Check sheet for the modelled part. Datum: model origin and axes. Units: mm. Face numbers are marked on the shaded views. A direction names the side the tool comes from. Coordinates: 2 decimals unless noted, no trailing zeros. Loops run counter-clockwise (first coordinate to the right, second up) from the corner with the lowest first, then second, coordinate; pieces in that order, holes last. Notation, with made-up numbers: (-20, 12.25) - (11, 12.25) arc R10 cw to (11, 19.25) - close; hole circle Ø4 at (-3.5, 45). An arc over 180 degrees is marked (long way). Use a Markdown table: item, result. Add a question column.
1) Draft check along X on the marked faces 6, 7 and 8. Enter one of: pulls with the +X half, pulls with the -X half, needs draft (parallel to the pull), parting line crosses it, or undercut.
2) Sectioned sample at C-C, the plane x = 8.5. Enter the section's corners in (y, z).
3) Go/stop test with flat-tipped pins: P1, Ø1.5, axis at x = 9, y = 47.5, coming from the -Z side; P2, Ø6, axis at x = 15, z = 42, coming from the +Y side; P3, Ø6, axis at y = 72.5, z = 7.5, coming from the -X side. Record where each tip stops, or that it passes through.
4) Sectioned sample at B-B, the plane y = 18. Enter the section's corners in (x, z), then the cut area to 3 significant figures.
5) Sectioned sample at D-D, the plane z = 7.5. Enter the section's corners in (x, y).
6) Thickness scan on line 1 (Y direction, x = 13.5, z = 55.5); line 2 (X direction, y = 2.55, z = 62.5); line 3 (X direction, y = 77.5, z = 4.5). Record the ranges inside material, lowest first.
7) Sectioned sample at A-A, the plane z = 62.5. Enter the section's corners in (x, y), then the cut area to 3 significant figures.
8) Tool access check on the marked faces 1, 2, 3, 4 and 5. Record the directions out of +Z, -Z, +X, -X, +Y, -Y that give a thin tool (end or side, any length) a straight path to the whole face; none if there is none.
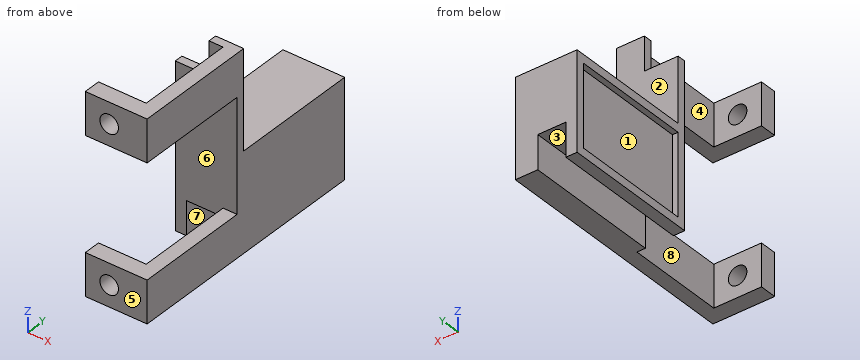
from build123d import *

# Parameters (mm, degrees)
SKETCH001_W  = 41
SKETCH001_H  = 40
PAD001_DEPTH = 22
SKETCH002_W  = 46
SKETCH002_H  = 35
PAD002_DEPTH = 22
SKETCH003_W  = 35
SKETCH003_H  = 17
PAD003_DEPTH = 70
SKETCH004_W  = 43
SKETCH004_H  = 29
PAD004_DEPTH = 2
SKETCH008_R  = 3.3
PAD006_DEPTH = 6
SKETCH007_R  = 3.3
PAD005_DEPTH = 6
SKETCH009_W  = 12
SKETCH009_H  = 12
PAD007_DEPTH = 3
SKETCH010_W  = 10
SKETCH010_H  = 49
PAD008_DEPTH = 12
SKETCH_W     = 90
SKETCH_H     = 70
PAD_DEPTH    = 22


with BuildPart() as body001:
    # Sketch001 (on Face1 of CopyPad) → Pad001 (new body)
    with BuildSketch(Plane.YZ.offset(22)):
        with Locations((20.5, 35)):
            Rectangle(SKETCH001_W, SKETCH001_H)
    extrude(amount=-PAD001_DEPTH)


with BuildPart() as body002:
    # Sketch002 (on Face1 of CopyPad001) → Pad002 (new body)
    with BuildSketch(Plane.YZ.offset(22)):
        with Locations((67, 52.5)):
            Rectangle(SKETCH002_W, SKETCH002_H)
    extrude(amount=-PAD002_DEPTH)


with BuildPart() as body003:
    # Sketch003 (on Face1 of CopyBoolean001) → Pad003 (new body)
    with BuildSketch(Plane.YX):
        with Locations((23.5, 8.5)):
            Rectangle(SKETCH003_W, SKETCH003_H)
    extrude(amount=-PAD003_DEPTH)


with BuildPart() as body004:
    # Sketch004 (on Face1 of CopyBoolean002) → Pad004 (new body)
    with BuildSketch(Plane(origin=(0, 0, 0), x_dir=(0, -1, 0), z_dir=(-1, 0, 0))):
        with Locations((-65.5, 17.5)):
            Rectangle(SKETCH004_W, SKETCH004_H)
    extrude(amount=-PAD004_DEPTH)


with BuildPart() as body007:
    # Sketch008 → Pad006 (new body)
    with BuildSketch(Plane(origin=(0, 0, 0), x_dir=(0, 0, -1), z_dir=(0, -1, 0))):
        with Locations((-7.5, 8.5)):
            Circle(SKETCH008_R)
    extrude(amount=-PAD006_DEPTH)


with BuildPart() as body007_1:
    # Body007 placement: moved
    add(body007.part.moved(Location((0, 0, 55))))


with BuildPart() as body006:
    # Sketch007 → Pad005 (new body)
    with BuildSketch(Plane(origin=(0, 0, 0), x_dir=(0, 0, -1), z_dir=(0, -1, 0))):
        with Locations((-7.5, 8.5)):
            Circle(SKETCH007_R)
    extrude(amount=-PAD005_DEPTH)


with BuildPart() as body008:
    # Sketch009 (on Face1 of CopyBoolean005) → Pad007 (new body)
    with BuildSketch(Plane.XZ.offset(-41)):
        with Locations((6, 64)):
            Rectangle(SKETCH009_W, SKETCH009_H)
    extrude(amount=-PAD007_DEPTH)


with BuildPart() as body009:
    # Sketch010 (on Face1 of CopyBoolean006) → Pad008 (new body)
    with BuildSketch(Plane(origin=(0, 0, 0), x_dir=(1, 0, 0), z_dir=(0, 0, -1))):
        with Locations((9, -65.5)):
            Rectangle(SKETCH010_W, SKETCH010_H)
    extrude(amount=-PAD008_DEPTH)


with BuildPart() as body:
    # Sketch → Pad (new body)
    with BuildSketch(Plane.YZ):
        with Locations((45, 35)):
            Rectangle(SKETCH_W, SKETCH_H)
    extrude(amount=PAD_DEPTH)

    # Boolean: cut Body001
    add(body001.part, mode=Mode.SUBTRACT)

    # Boolean001: cut Body002
    add(body002.part, mode=Mode.SUBTRACT)

    # Boolean002: cut Body003
    add(body003.part, mode=Mode.SUBTRACT)

    # Boolean003: cut Body004
    add(body004.part, mode=Mode.SUBTRACT)

    # Boolean004: cut Body007
    add(body007_1.part, mode=Mode.SUBTRACT)

    # Boolean005: cut Body006
    add(body006.part, mode=Mode.SUBTRACT)

    # Boolean006: cut Body008
    add(body008.part, mode=Mode.SUBTRACT)

    # Boolean007: cut Body009
    add(body009.part, mode=Mode.SUBTRACT)


solid = body.part
Solved:
| question | item | result |
|---|---|---|
| 1 | face 6 | needs draft |
| 1 | face 7 | undercut |
| 1 | face 8 | pulls with the -X half |
| 2 | outline | (0, 0) - (6, 0) - (6, 4.2) - (0, 4.2) - close; (0, 10.8) - (6, 10.8) - (6, 15) - (0, 15) - close; (0, 55) - (6, 55) - (6, 59.2) - (0, 59.2) - close; (0, 65.8) - (6, 65.8) - (6, 70) - (0, 70) - close; (41, 12) - (90, 12) - (90, 35) - (44, 35) - (44, 58) - (41, 58) - close |
| 3 | P1 | stops at z = 12 |
| 3 | P2 | stops at y = 44 |
| 3 | P3 | stops at x = 2 |
| 4 | outline | (17, 0) - (22, 0) - (22, 15) - (17, 15) - close; (17, 55) - (22, 55) - (22, 70) - (17, 70) - close |
| 4 | area | 150 mm2 |
| 5 | outline | (0, 0) - (5.2, 0) - (5.2, 6) - (0, 6) - close; (0, 41) - (4, 41) - (4, 90) - (0, 90) - (0, 87) - (2, 87) - (2, 44) - (0, 44) - close; (11.8, 0) - (22, 0) - (22, 90) - (14, 90) - (14, 41) - (17, 41) - (17, 6) - (11.8, 6) - close |
| 6 | line 1 | y = 0 to 6, 41 to 44 |
| 6 | line 2 | x = 0 to 5.2, 11.8 to 22 |
| 6 | line 3 | x = 2 to 4, 14 to 22 |
| 7 | outline | (0, 0) - (5.2, 0) - (5.2, 6) - (0, 6) - close; (11.8, 0) - (22, 0) - (22, 44) - (12, 44) - (12, 41) - (17, 41) - (17, 6) - (11.8, 6) - close |
| 7 | area | 297 mm2 |
| 8 | face 1 | -X |
| 8 | face 2 | +Z, +X, -X, +Y |
| 8 | face 3 | -Z, +Y |
| 8 | face 4 | +Z, -Z, -X |
| 8 | face 5 | +Z, -Z, +X, -X, -Y |
